Read the model definition and answer for the solid it produces. Units are mm, in the model's axes. A direction names the side the tool comes from. Round coordinates to 2 decimals unless told otherwise and drop trailing zeros. Loops run counter-clockwise (first coordinate to the right, second up) from the corner with the lowest first, then second, coordinate; pieces in that order, holes last. Notation, with made-up numbers: M 31.5,51 L 87.5,51 A15 ccw 87.5,78 Z; hole C 45,27 d9. An arc over 180 degrees is marked long. Write each question's results on one line, items separated by ' | '.
Autodesk Fusion 360 part; units mm, degrees
sketch "Sketch1" plane through (0, 0, 0) normal (0, 0, 1) x (1, 0, 0)
  line L0 (0, 3.5) -> (40, 3.5)
  line L1 (40, 3.5) -> (40, -3.5)
  line L2 (40, -3.5) -> (0, -3.5)
  line L3 (0, -3.5) -> (0, 3.5)
  line L4 (0, 3.5) -> (7, 3.5)
  line L5 (7, 3.5) -> (7, -3.5)
  line L6 (7, -3.5) -> (0, -3.5)
  line L7 (0, -3.5) -> (0, 3.5)
  line L8 (40, 3.5) -> (19, 3.5)
  line L9 (19, 3.5) -> (19, -3.5)
  line L10 (19, -3.5) -> (40, -3.5)
  line L11 (40, -3.5) -> (40, 3.5)
  dimension "d1" = 7
  dimension "d2" = 40
  dimension "d5" = 7
  dimension "d14" = 21
  dimension "d19" = 34
extrude "Extrude3" add sketch "Sketch1" along normal blind 9 contours L0 L2 L5 L9 makes body 1
extrude "Extrude2" add sketch "Sketch1" along normal blind 20 separate body contours L0 L2 L3 L4 L5 L6 L7 makes body 2
extrude "Extrude1" add sketch "Sketch1" along normal blind 2.8 bodies 1 2
fillet "Fillet3" radius 2 6 edges at (7, -3.5, 14.5) (0, -3.5, 10) (0, 3.5, 10) (7, 3.5, 14.5) (40, 3.5, 1.4) (40, -3.5, 1.4) on bodies 1
fillet "Fillet4" radius 1 8 edges at (6.4142, -2.9142, 20) (7, 0, 20) (6.4142, 2.9142, 20) (3.5, 3.5, 20) (0.5858, 2.9142, 20) (0, 0, 20) (0.5858, -2.9142, 20) (3.5, -3.5, 20) on bodies 1
Item 1: The part is cut by section A-A (y = -0.25). Determine the outline of the cut face in (x, z).
Outcome:
outline: M 0,0 L 40,0 L 40,2.8 L 19,2.8 L 19,9 L 7,9 L 7,19 A1 ccw 6,20 L 1,20 A1 ccw 0,19 Z
Item 2: For faces 1 (the face through (3, 0, 20)), 2 (the face through (6.43, 2.9, 14.07)), 3 (the face through (6.4, -2.93, 14.07)), 4 (the face through (0.6, -2.93, 9.37)), 5 (the face through (7, 0, 14)), determine the directions among +Z, -Z, +X, -X, +Y, -Y from which every point of the face is accessible in a straight line to the end or side of a thin tool.
Outcome:
face 1: +Z, +X, -X, +Y, -Y | face 2: +Z, +X, +Y | face 3: +Z, +X, -Y | face 4: +Z, -Z, -X, -Y | face 5: +Z, +X, +Y, -Y
Item 3: Straight lines are drawn through the part: line 1 (X direction, y = 0.75, z = 4.25); line 2 (Z direction, x = 33.5, y = -3); line 3 (Z direction, x = 12.5, y = -2.5). For each, find the intervals that lie inside material, in ascending order.
Outcome:
line 1: x = 0 to 19 | line 2: z = 0 to 2.8 | line 3: z = 0 to 9
Item 4: The part is cut by section D-D (x = 17.5). Determine the outline of the cut face in (y, z).
Outcome:
outline: M -3.5,0 L 3.5,0 L 3.5,9 L -3.5,9 Z
Item 5: Flat-ended cylindrical pins translate along their axes: pin 1 (3.5 mm diameter, centred on x = 13, y = 0, fed in from +Z); pin 2 (1.5 mm diameter, centred on y = 0.5, z = 5.5, fed in from +X); pin 3 (2 mm diameter, centred on x = 28.5, y = -1, fed in from +Z). Find the tip coordinate at first contact, or state that the pin passes through.
Outcome:
pin 1: stops at z = 9 | pin 2: stops at x = 19 | pin 3: stops at z = 2.8
Item 6: The part is cut by section B-B (z = 16.5). Determine the outline of the cut face in (x, y), plus the area to 3 significant figures.
Outcome:
outline: M 0,-1.5 A2 ccw 2,-3.5 L 5,-3.5 A2 ccw 7,-1.5 L 7,1.5 A2 ccw 5,3.5 L 2,3.5 A2 ccw 0,1.5 Z | area: 45.6 mm2
Item 7: The part is cut by section C-C (x = 24.5). Determine the outline of the cut face in (y, z), plus the area to 3 significant figures.
Outcome:
outline: M -3.5,0 L 3.5,0 L 3.5,2.8 L -3.5,2.8 Z | area: 19.6 mm2
